from build123d import *

# Parameters (mm, degrees)
SKETCH1_R           = 2.4892
SKETCH1_R_2         = 2.9718
BOSS_EXTRUDE1_DEPTH = 3.175
SKETCH2_W           = 18.4277
SKETCH2_H           = 6.35
CUT_EXTRUDE1_DEPTH  = 4.175


with BuildPart() as part:
    # Sketch1 → Boss-Extrude1 (new body)
    with BuildSketch(Plane.XY):
        Polygon((37.4777, 9.5377), (0, 9.5377), (0, 3.1877), (18.4277, 3.1877), (18.4277, -19.0373), (0, -19.0373), (0, -25.3873), (12.0777, -25.3873), (12.0777, -41.2623), (37.4777, -41.2623), align=None)
        with Locations((23.471581917, -33.3248)):
            Circle(SKETCH1_R, mode=Mode.SUBTRACT)
        with Locations((23.471581917, -7.9248)):
            Circle(SKETCH1_R_2, mode=Mode.SUBTRACT)
    extrude(amount=BOSS_EXTRUDE1_DEPTH)

    # Sketch2 → Cut-Extrude1 (cut, through all)
    with BuildSketch(Plane(origin=(0, 0, 0), x_dir=(-1, 0, 0), z_dir=(0, 0, -1))):
        with Locations((-9.21385, 6.3627)):
            Rectangle(SKETCH2_W, SKETCH2_H)
    extrude(amount=-CUT_EXTRUDE1_DEPTH, mode=Mode.SUBTRACT)


solid = part.part
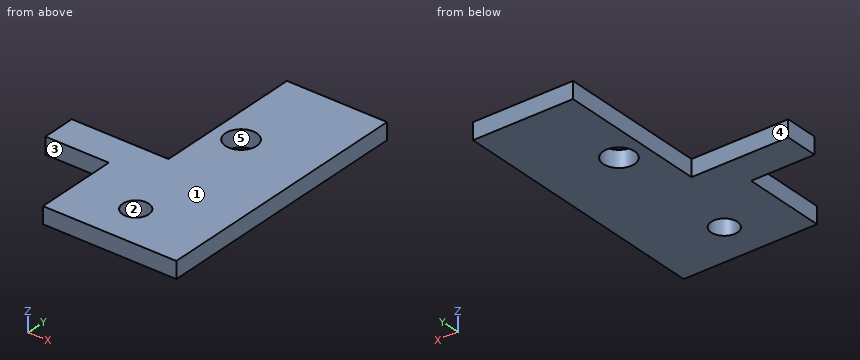
Geometry: final body of the model. Coordinates: model frame, mm. Face numbers are marked on the shaded views. A direction names the side the tool comes from. Coordinates: 2 decimals unless noted, no trailing zeros. Order: outer loops, then holes, each group sorted by start corner. A loop starts at its lowest first (then second) coordinate and runs counter-clockwise, first axis right, second up.
(1) Section query D-D (x = 13.5). Return the cut outline in (y, z) (3 decimals), plus the area to 3 significant figures.
(2) Access query for the marked faces 4 and 5. Directions: +Z, -Z, +X, -X, +Y, -Y. A direction counts if a zero-diameter tool reaches every point of the face in a straight line with its end or side. Return the directions, or none.
(3) Draft query along Y for the marked faces 1, 2 and 3. Return one class per face: pulls with the +Y half, pulls with the -Y half, needs draft (parallel to the pull), parting line crosses it, or undercut.
(4) First-contact query: pin 1 (1.6 mm diameter, centred on y = -7.5, z = 1, fed in from -X); pin 2 (1 mm diameter, centred on x = 7.5, z = 1, fed in from -Y); pin 3 (1 mm diameter, centred on y = -37, z = 1, fed in from -X). Flat tips, straight axial feed; report the tip coordinate or a pass-through.
(5) Section query C-C (y = -36.5). Return the cut outline in (x, z) (3 decimals), plus the area to 3 significant figures.
(6) Material intervals for probe 1 along X at (y, z) = (-1, 2); probe 2 along X at (y, z) = (-29, 0.9); probe 3 along X at (y, z) = (-34, 0.65), sorted ascending.
(7) Section query A-A (y = -5.5). Return the cut outline in (x, z) (3 decimals), plus the area to 3 significant figures.
(8) Section query B-B (z = 2.4). Return the cut outline in (x, y), plus the area to 3 significant figures.
Solution:
1. outline: (-41.262, 0) - (-19.037, 0) - (-19.037, 3.175) - (-41.262, 3.175) - close
1. area: 70.6 mm2
2. face 4: +Z, -Z, -X, +Y
2. face 5: +Z, -Z
3. face 1: needs draft
3. face 2: undercut
3. face 3: pulls with the -Y half
4. pin 1: stops at x = 18.43
4. pin 2: stops at y = -25.39
4. pin 3: stops at x = 12.08
5. outline: (12.078, 0) - (37.478, 0) - (37.478, 3.175) - (12.078, 3.175) - close
5. area: 80.6 mm2
6. probe 1: x = 18.43 to 37.48
6. probe 2: x = 12.08 to 37.48
6. probe 3: x = 12.08 to 21.08, 25.87 to 37.48
7. outline: (18.428, 0) - (21.753, 0) - (21.753, 3.175) - (18.428, 3.175) - close; (25.19, 0) - (37.478, 0) - (37.478, 3.175) - (25.19, 3.175) - close
7. area: 49.6 mm2
8. outline: (0, -25.39) - (12.08, -25.39) - (12.08, -41.26) - (37.48, -41.26) - (37.48, 9.54) - (18.43, 9.54) - (18.43, -19.04) - (0, -19.04) - close; hole circle Ø5.94 at (23.47, -7.92); hole circle Ø4.98 at (23.47, -33.32)
8. area: 1,140 mm2
